For this review, take the finished solid that the model builds, in its own axes (mm). Give positions to 0.01 mm unless a question says otherwise; leave off trailing zeros. Order: outer loops, then holes, each group sorted by start corner. A loop starts at its lowest first (then second) coordinate and runs counter-clockwise, first axis right, second up.
Item 1: Consider section C-C (x = -52). Give the boundary of the cut face in (y, z).
Item 2: Consider section D-D (y = 4.75). Give the number of separate pieces and of enclosed holes in the cut face, plus the area to 3 significant figures.
Item 3: Consider section B-B (y = 12.5). Give the boundary of the cut face in (x, z), plus the area to 3 significant figures.
Item 4: For probe 1 along Z at (x, y) = (-51, 2.75); probe 2 along Z at (x, y) = (-47.5, 12.25); probe 3 along X at (y, z) = (12.5, 27.5), list the stretches that pass through material, from the lowest coordinate up.
Item 5: For P1, Ø6, axis at x = -10, z = -32.5, coming from the +Y side; P2, Ø2, axis at x = -50, y = 7, coming from the -Z side; P3, Ø2.5, axis at y = 12, z = 27.5, coming from the -X side, all flat-tipped, find the tip position at first contact; note any pin that passes through.
Item 6: Consider section A-A (z = -38). Give the boundary of the cut face in (x, y).
```python
from build123d import *

# Parameters (mm, degrees)
SKETCH1_W           = 58
SKETCH1_H           = 75
BOSS_EXTRUDE1_DEPTH = 8.5
SKETCH4_R           = 3
CUT_EXTRUDE1_DEPTH  = 6.5
SKETCH5_W           = 12
SKETCH5_H           = 12
BOSS_EXTRUDE2_DEPTH = 5
SKETCH8_W           = 2
SKETCH8_H           = 8.5
BOSS_EXTRUDE3_DEPTH = 2
SKETCH7_W           = 8
SKETCH7_H           = 7
BOSS_EXTRUDE4_DEPTH = 12
SKETCH9_R           = 1.95
CUT_EXTRUDE2_DEPTH  = 7
FILLET1_R           = 4


with BuildPart() as part:
    # Sketch1 → Boss-Extrude1 (new body)
    with BuildSketch(Plane(origin=(0, 0, 0), x_dir=(1, 0, 0), z_dir=(0, 1, 0))):
        with Locations((-28.734265734, -3.094405594)):
            Rectangle(SKETCH1_W, SKETCH1_H)
    extrude(amount=BOSS_EXTRUDE1_DEPTH)

    # Sketch4 → Cut-Extrude1 (cut)
    # profile 1 of 4: a face of its own
    with BuildSketch(Plane(origin=(0, 8.5, 0), x_dir=(1, 0, 0), z_dir=(0, 1, 0))):
        with BuildLine():
            Line((-57.734265734, 7.605594406), (-57.734265734, 5.105594406))
            Line((-57.734265734, 5.105594406), (-47.937319909, 5.105594406))
            ThreePointArc((-47.937319909, 5.105594406), (-46.897035131, 4.919454313), (-45.985842823, 4.384132793))
            Line((-45.985842823, 4.384132793), (-42.13114507, 1.082738189))
            ThreePointArc((-42.13114507, 1.082738189), (-34.749045592, 3.244128144), (-40.069670138, 8.799121725))
            Line((-40.069670138, 8.799121725), (-45.137956932, 7.676576192))
            ThreePointArc((-45.137956932, 7.676576192), (-45.46038672, 7.623392649), (-45.786688237, 7.605594406))
            Line((-45.786688237, 7.605594406), (-57.734265734, 7.605594406))
        make_face()
        with Locations(Location((-39.096573179, 4.405594406, 0), (0, 0, 270))):
            Circle(SKETCH4_R, mode=Mode.SUBTRACT)
    # profile 2 of 4: a face of its own
    with BuildSketch(Plane(origin=(0, 8.5, 0), x_dir=(1, 0, 0), z_dir=(0, 1, 0))):
        with BuildLine():
            Line((-57.734265734, -13.794405594), (-57.734265734, -11.294405594))
            Line((-57.734265734, -11.294405594), (-47.937319909, -11.294405594))
            ThreePointArc((-47.937319909, -11.294405594), (-46.897035131, -11.108265502), (-45.985842823, -10.572943982))
            Line((-45.985842823, -10.572943982), (-42.13114507, -7.271549377))
            ThreePointArc((-42.13114507, -7.271549377), (-34.749045592, -9.432939333), (-40.069670138, -14.987932914))
            Line((-40.069670138, -14.987932914), (-45.137956932, -13.865387381))
            ThreePointArc((-45.137956932, -13.865387381), (-45.46038672, -13.812203837), (-45.786688237, -13.794405594))
            Line((-45.786688237, -13.794405594), (-57.734265734, -13.794405594))
        make_face()
        with Locations(Location((-39.096573179, -10.594405594, 0), (0, 0, 270))):
            Circle(SKETCH4_R, mode=Mode.SUBTRACT)
    # profile 3 of 4: a face of its own
    with BuildSketch(Plane(origin=(0, 8.5, 0), x_dir=(1, 0, 0), z_dir=(0, 1, 0))):
        with BuildLine():
            Line((0.265734266, -13.794405594), (0.265734266, -11.294405594))
            Line((0.265734266, -11.294405594), (-9.531211559, -11.294405594))
            ThreePointArc((-9.531211559, -11.294405594), (-10.571496337, -11.108265502), (-11.482688645, -10.572943982))
            Line((-11.482688645, -10.572943982), (-15.337386398, -7.271549377))
            ThreePointArc((-15.337386398, -7.271549377), (-22.719485877, -9.432939333), (-17.39886133, -14.987932914))
            Line((-17.39886133, -14.987932914), (-12.330574537, -13.865387381))
            ThreePointArc((-12.330574537, -13.865387381), (-12.008144749, -13.812203837), (-11.681843231, -13.794405594))
            Line((-11.681843231, -13.794405594), (0.265734266, -13.794405594))
        make_face()
        with Locations(Location((-18.371958289, -10.594405594, 0), (0, 0, 270))):
            Circle(SKETCH4_R, mode=Mode.SUBTRACT)
    # profile 4 of 4: a face of its own
    with BuildSketch(Plane(origin=(0, 8.5, 0), x_dir=(1, 0, 0), z_dir=(0, 1, 0))):
        with BuildLine():
            Line((0.265734266, 7.605594406), (0.265734266, 5.105594406))
            Line((0.265734266, 5.105594406), (-9.531211559, 5.105594406))
            ThreePointArc((-9.531211559, 5.105594406), (-10.571496337, 4.919454313), (-11.482688645, 4.384132793))
            Line((-11.482688645, 4.384132793), (-15.337386398, 1.082738189))
            ThreePointArc((-15.337386398, 1.082738189), (-22.719485877, 3.244128144), (-17.39886133, 8.799121725))
            Line((-17.39886133, 8.799121725), (-12.330574537, 7.676576192))
            ThreePointArc((-12.330574537, 7.676576192), (-12.008144749, 7.623392649), (-11.681843231, 7.605594406))
            Line((-11.681843231, 7.605594406), (0.265734266, 7.605594406))
        make_face()
        with Locations(Location((-18.371958289, 4.405594406, 0), (0, 0, 270))):
            Circle(SKETCH4_R, mode=Mode.SUBTRACT)
    extrude(amount=-CUT_EXTRUDE1_DEPTH, mode=Mode.SUBTRACT)

    # Sketch5 → Boss-Extrude2 (add)
    with BuildSketch(Plane(origin=(0, 8.5, 0), x_dir=(1, 0, 0), z_dir=(0, 1, 0))):
        with Locations((-41.734265734, 18.405594406)):
            Rectangle(SKETCH5_W, SKETCH5_H)
        with Locations((-15.734265734, 18.405594406)):
            Rectangle(SKETCH5_W, SKETCH5_H)
        with Locations((-15.734265734, -24.594405594)):
            Rectangle(SKETCH5_W, SKETCH5_H)
        with Locations((-41.734265734, -24.594405594)):
            Rectangle(SKETCH5_W, SKETCH5_H)
    extrude(amount=BOSS_EXTRUDE2_DEPTH)

    # Sketch8 → Boss-Extrude3 (add)
    with BuildSketch(Plane(origin=(0, 0, -34.405594406), x_dir=(-1, 0, 0), z_dir=(0, 0, -1))):
        with Locations((37.734265734, 4.25)):
            Rectangle(SKETCH8_W, SKETCH8_H)
        with Locations((19.734265734, 4.25)):
            Rectangle(SKETCH8_W, SKETCH8_H)
    extrude(amount=BOSS_EXTRUDE3_DEPTH)

    # Sketch7 → Boss-Extrude4 (add)
    with BuildSketch(Plane(origin=(0, 0, -34.405594406), x_dir=(-1, 0, 0), z_dir=(0, 0, -1))):
        with Locations((45.734265734, 3.5)):
            Rectangle(SKETCH7_W, SKETCH7_H)
        with Locations((11.734265734, 3.5)):
            Rectangle(SKETCH7_W, SKETCH7_H)
    extrude(amount=BOSS_EXTRUDE4_DEPTH)

    # Sketch9 → Cut-Extrude2 (cut)
    with BuildSketch(Plane(origin=(0, 0, 0), x_dir=(-1, 0, 0), z_dir=(0, -1, 0))):
        with Locations(Location((11.734265734, 41.405594406, 0), (0, 0, 90))):
            Circle(SKETCH9_R)
        with Locations(Location((45.734265734, 41.405594406, 0), (0, 0, 90))):
            Circle(SKETCH9_R)
    extrude(amount=-CUT_EXTRUDE2_DEPTH, mode=Mode.SUBTRACT)

    # Fillet1
    fillet1_edges = [part.edges().sort_by_distance(p)[0] for p in [
        (-7.734265734, 3.5, -46.405594406),
        (-15.734265734, 3.5, -46.405594406),
        (-49.734265734, 3.5, -46.405594406),
        (-41.734265734, 3.5, -46.405594406),
    ]]
    fillet(fillet1_edges, radius=FILLET1_R - 0.0001)  # a hair under: the kernel refuses the full size


solid = part.part
```
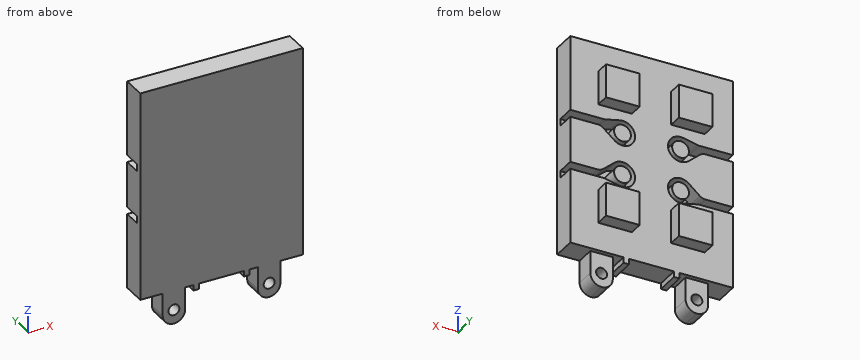
Resolved:
1. outline: (0, -34.41) - (8.5, -34.41) - (8.5, -7.61) - (2, -7.61) - (2, -5.11) - (8.5, -5.11) - (8.5, 11.29) - (2, 11.29) - (2, 13.79) - (8.5, 13.79) - (8.5, 40.59) - (0, 40.59) - close
2. separate pieces: 5
2. enclosed holes: 2
2. area: 4,200 mm2
3. outline: (-47.73, -24.41) - (-35.73, -24.41) - (-35.73, -12.41) - (-47.73, -12.41) - close; (-47.73, 18.59) - (-35.73, 18.59) - (-35.73, 30.59) - (-47.73, 30.59) - close; (-21.73, -24.41) - (-9.73, -24.41) - (-9.73, -12.41) - (-21.73, -12.41) - close; (-21.73, 18.59) - (-9.73, 18.59) - (-9.73, 30.59) - (-21.73, 30.59) - close
3. area: 576 mm2
4. probe 1: z = -34.41 to -7.61, -5.11 to 11.29, 13.79 to 40.59
4. probe 2: z = -24.41 to -12.41, 18.59 to 30.59
4. probe 3: x = -47.73 to -35.73, -21.73 to -9.73
5. P1: stops at y = 8.5
5. P2: stops at z = -44.72
5. P3: stops at x = -47.73
6. outline: (-49.73, 0) - (-41.73, 0) - (-41.73, 7) - (-49.73, 7) - close; (-15.73, 0) - (-7.73, 0) - (-7.73, 7) - (-15.73, 7) - close
